Study the drawing (mm; zero at the part's minimum x, y, z) and answer. A direction names the side the tool comes from. Round coordinates to 2 decimals unless told otherwise and drop trailing zeros. Write each loop counter-clockwise with the first axis right and the second up, starting at its lowest first coordinate (ties: lowest second). Pieces come first, ordered by that corner, then holes. Notation, with made-up numbers: M 30,82.5 L 50,82.5 A15 cw 50,94.5 Z; hole C 66.25,84 d4. An arc over 180 degrees is marked long. Write each question's results on one line, items separated by ' | '.
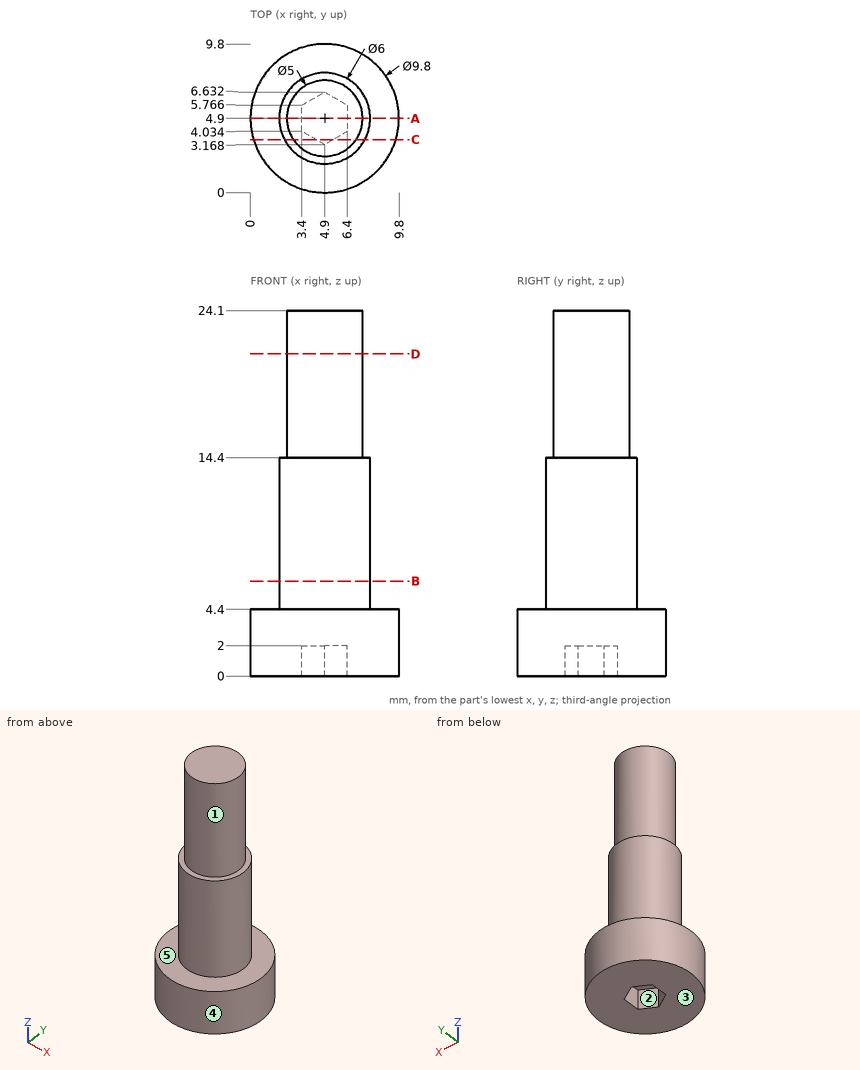
1) Section A-A (y = 4.9) is taken. Determine the outline of the cut face in (x, z).
Return value:
outline: M 0,0 L 3.4,0 L 3.4,2 L 6.4,2 L 6.4,0 L 9.8,0 L 9.8,4.4 L 7.9,4.4 L 7.9,14.4 L 7.4,14.4 L 7.4,24.1 L 2.4,24.1 L 2.4,14.4 L 1.9,14.4 L 1.9,4.4 L 0,4.4 Z
2) Find the intervals of material crossed by line 1 (Z direction, x = 1, y = 5.25); line 2 (Z direction, x = 5.5, y = 5.25); line 3 (Y direction, x = 6.25, z = 8.5), in increasing order.
Return value:
line 1: 0 to 4.4 | line 2: 2 to 24.1 | line 3: 2.22 to 7.58
3) Section B-B (z = 6.25) is taken. Determine the outline of the cut face in (x, y).
Return value:
outline: C 4.9,4.9 d6
4) Each of these flat-tipped pins is pushed along its axis until it touches: pin 1 (2 mm diameter, centred on x = 1.5, y = 2.5, fed in from +Z); pin 2 (4 mm diameter, centred on x = 7, z = 11.5, fed in from -Y); pin 3 (4 mm diameter, centred on x = 2.5, z = 21, fed in from -Y). Where does it stop, or does it pass through?
Return value:
pin 1: z = 4.4 | pin 2: y = 1.9 | pin 3: y = 2.43
5) A tool of negligible diameter and unlimited length cuts with its end or side. For the marked faces 4 and 5, from which of +Z, -Z, +X, -X, +Y, -Y can it reach the whole face along a straight path? Write none if from no direction.
Return value:
face 4: +Z, -Z | face 5: +Z
6) The mould has two halves that part along X. Classify the marked faces 1, 2 and 3: +X half, -X half, draft (parallel to the pull), parting line (faces both ways), or undercut.
Return value:
face 1: parting line | face 2: undercut | face 3: draft
7) Section C-C (y = 3.5) is taken. Determine the outline of the cut face in (x, z).
Return value:
outline: M 0.2,0 L 4.32,0 L 4.32,2 L 5.48,2 L 5.48,0 L 9.6,0 L 9.6,4.4 L 7.55,4.4 L 7.55,14.4 L 6.97,14.4 L 6.97,24.1 L 2.83,24.1 L 2.83,14.4 L 2.25,14.4 L 2.25,4.4 L 0.2,4.4 Z
8) Section D-D (z = 21.25) is taken. Determine the outline of the cut face in (x, y), then the cut area to 3 significant figures.
Return value:
outline: C 4.9,4.9 d5 | area: 19.6 mm²
